```python
from build123d import *

# Parameters (mm, degrees)
F2_W      = 50.8
F2_H      = 38.1
F4_W      = 101.6
F4_H      = 38.1
F5_DEPTH  = 76.2010001
F6_W      = 38.1
F6_H      = 38.1
F7_DEPTH  = 7.62
F8_R      = 6.35
F9_DEPTH  = 20.32
F9_TAPER  = -40
F10_R     = 6.35
F11_DEPTH = 25.4
F12_R     = 3.81
F13_DEPTH = 33.02


with BuildPart() as f1:
    # F0 (on Front) → F1 (revolve)
    with BuildSketch(Plane.XZ):
        with BuildLine():
            Line((0, 0), (76.2, 0))
            add(Edge.make_bspline(
                [(76.2, 0), (76.2, 30.4536055773), (76.2, 58.42), (63.5, 58.42)],
                knots=[0, 0, 0, 0, 59.7844996634, 59.7844996634, 59.7844996634, 59.7844996634], degree=3))
            Line((63.5, 58.42), (0, 58.42))
            Line((0, 58.42), (0, 0))
        make_face()
    revolve(axis=Axis((0, 0, 29.21), (0, 0, 1)))

    # F2 (on Front) → F3 (revolve, cut)
    with BuildSketch(Plane.XZ):
        with Locations((25.4, 31.75)):
            Rectangle(F2_W, F2_H)
    revolve(axis=Axis((0, 0, 31.75), (0, 0, 1)), mode=Mode.SUBTRACT)

    # F4 (on Front) → F5 (cut, through all)
    with BuildSketch(Plane.XZ):
        with Locations((0, 31.75)):
            Rectangle(F4_W, F4_H)
    extrude(amount=F5_DEPTH, mode=Mode.SUBTRACT)

    # F6 (on face) → F7 (join)
    with BuildSketch(Plane(origin=(0, 0, 0), x_dir=(1, 0, 0), z_dir=(0, 0, -1))):
        Rectangle(F6_W, F6_H)
    extrude(amount=F7_DEPTH)

    # F8 (on face) → F9 (cut, through all)
    with BuildSketch(Plane(origin=(0, 0, -7.62), x_dir=(1, 0, 0), z_dir=(0, 0, -1))):
        Circle(F8_R)
    extrude(amount=-F9_DEPTH, taper=F9_TAPER, mode=Mode.SUBTRACT)

    # F10 (on face) → F11 (join)
    with BuildSketch(Plane.XY.offset(58.42)):
        Circle(F10_R)
    extrude(amount=F11_DEPTH)

    # F12 (on face) → F13 (cut, through all)
    with BuildSketch(Plane.XY.offset(83.82)):
        Circle(F12_R)
    extrude(amount=-F13_DEPTH, mode=Mode.SUBTRACT)


solid = f1.part
```
Can you work these out from the model? Positions are in its coordinate system, mm. A direction names the side the tool comes from. Coordinates: 2 decimals unless noted, no trailing zeros. Loops run counter-clockwise (first coordinate to the right, second up) from the corner with the lowest first, then second, coordinate; pieces in that order, holes last. Notation, with made-up numbers: (-27.75, 83.25) -> (13.25, 83.25) arc R18 cw to (13.25, 95.25) -> close; hole circle Ø5 at (63, 26). An arc over 180 degrees is marked (long way). Put each result on its own line as item: value. Start each with the question number.
Q1. I'm going to push flat-ended pins straight in: P1, Ø1.5, axis at x = 38, z = 8, coming from the -Y side; P2, Ø8, axis at y = 20.5, z = 25.5, coming from the +X side; P3, Ø11.5, axis at y = -24.5, z = 34.5, coming from the -X side; P4, Ø6, axis at x = 0, y = 0, coming from the -Z side. Where does each tip first touch, or does it pass through?
Q2. I want a section at B-B (z = 66). Write out the boundary of the cut face in (x, y), plus the area to 3 significant figures.
Q3. For faces 1 (the face through (19.05, 0, -4)), 2 (the face through (-50.8, -28, 31)), 3 (the face through (-1.212, -9.232, -4.091)), 4 (the face through (-19.05, 0, -4)), 5 (the face through (0, 19.05, -4)), which set-ups out of +Z, -Z, +X, -X, +Y, -Y let a thin tool reach every point of the face, with its end or its side?
Q4. Thinking about a two-plate mould opening in Z: for faces 6 (the face through (0, -19.05, -4)), 7 (the face through (50.8, -28, 31)), 8 (the face through (13, 1, 58.42)), 9 (the face through (-1, -26, 12.7)), which applies, pulls with the +Z half, pulls with the -Z half, needs draft (parallel to the pull), parting line crosses it, or undercut?
Q5. If I drill on line 1 (Z direction, x = -27.5, y = -45); line 2 (Y direction, x = 0, z = 63); line 3 (Y direction, x = -10.5, z = -3.5), over which ranges is the centre line in solid material (lowest first)? Write a range as [from, to].
Q6. I want a section at A-A (x = 0). Count the separate pieces of the cut face and the enclosed holes in it, plus the area to 3 significant figures.
Taken from the geometry:
1. P1: stops at y = -66.46
1. P2: stops at x = 74.08
1. P3: stops at x = -73.03
1. P4: passes through
2. outline: circle Ø12.7 at (0, 0); hole circle Ø7.62 at (0, 0)
2. area: 81.1 mm2
3. face 1: -Z, +X, +Y, -Y
3. face 2: -Y
3. face 3: none
3. face 4: -Z, -X, +Y, -Y
3. face 5: -Z, +X, -X, +Y
4. face 6: needs draft
4. face 7: undercut
4. face 8: pulls with the +Z half
4. face 9: undercut
5. line 1: z = [0, 12.7], [50.8, 58.42]
5. line 2: y = [-6.35, -3.81], [3.81, 6.35]
5. line 3: y = [-19.05, 19.05]
6. separate pieces: 3
6. enclosed holes: 0
6. area: 3,680 mm2
